Source: CAD feature listing. Evaluate the final solid. Frame: model axes, mm. Face numbers are marked on the shaded views. A direction names the side the tool comes from. Round coordinates to 2 decimals unless told otherwise and drop trailing zeros. Loops run counter-clockwise (first coordinate to the right, second up) from the corner with the lowest first, then second, coordinate; pieces in that order, holes last. Notation, with made-up numbers: (21, 40) - (42, 40) arc R18 cw to (42, 59) - close; hole circle Ø10 at (79.5, 74.25). An arc over 180 degrees is marked (long way). Use CSV: the item, a comma, the result in double quotes. Start each with the question number.
from build123d import *

# Parameters (mm, degrees)
BOSS_EXTRUDE1_DEPTH = 15
SKETCH2_W           = 5.5
SKETCH2_H           = 1.517546376


with BuildPart() as part:
    # Sketch1 → Boss-Extrude1 (new body)
    with BuildSketch(Plane.XY):
        with BuildLine():
            Line((-20, 0), (-20, 23))
            Line((-20, 23), (20, 23))
            Line((20, 23), (20, 0))
            Line((20, 0), (7.5, 0))
            ThreePointArc((7.5, 0), (0, 7.5), (-7.5, 0))
            Line((-7.5, 0), (-20, 0))
        make_face()
    extrude(amount=BOSS_EXTRUDE1_DEPTH)

    # Sketch2 → Cut-Revolve2 (revolve, cut)
    with BuildSketch(Plane(origin=(0, 0, 0), x_dir=(0, 0, -1), z_dir=(1, 0, 0))):
        with Locations((-7.5, 7.241226812)):
            Rectangle(SKETCH2_W, SKETCH2_H)
    revolve(axis=Axis((0, 0, 0), (0, 0, 1)), mode=Mode.SUBTRACT)


solid = part.part
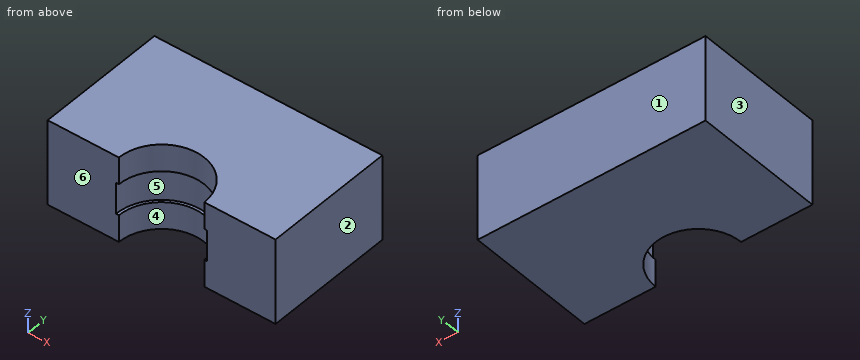
1. Section query D-D on x = 0. Return the cut outline in (y, z).
2. Section query A-A on y = 5.5. Return the cut outline in (x, z).
3. Line query: line 1 along X through (y, z) = (1.5, 12); line 2 along X through (y, z) = (5.5, 6.25); line 3 along Y through (x, z) = (5, 8.75) (3 decimals). Output: solid intervals per line, ascending.
4. Reachability of the marked faces 5 and 6 from +Z, -Z, +X, -X, +Y, -Y: full face, straight path, thin tool, end or side. Return the list, or none.
5. Mould query, pull axis X, two halves, no side actions, for the marked faces 1, 2, 3 and 4. Classes: +X half, -X half, draft (parallel to the pull), parting line (faces both ways), or undercut.
6. Section query C-C on x = 6. Return the cut outline in (y, z).
7. Section query B-B on z = 6. Return the cut outline in (x, y), and give its area (3 significant figures).
Values:
1,outline,"(7.5, 0) - (23, 0) - (23, 15) - (7.5, 15) - (7.5, 10.25) - (8, 10.25) - (8, 4.75) - (7.5, 4.75) - close"
2,outline,"(-20, 0) - (-5.1, 0) - (-5.1, 4.75) - (-5.81, 4.75) - (-5.81, 10.25) - (-5.1, 10.25) - (-5.1, 15) - (-20, 15) - close; (5.1, 0) - (20, 0) - (20, 15) - (5.1, 15) - (5.1, 10.25) - (5.81, 10.25) - (5.81, 4.75) - (5.1, 4.75) - close"
3,line 1,"x = -20 to -7.35, 7.35 to 20"
3,line 2,"x = -20 to -5.81, 5.81 to 20"
3,line 3,"y = 6.245 to 23"
4,face 5,"-Y"
4,face 6,"+Z, -Z, +X, -X, -Y"
5,face 1,"draft"
5,face 2,"+X half"
5,face 3,"-X half"
5,face 4,"undercut"
6,outline,"(4.5, 0) - (23, 0) - (23, 15) - (4.5, 15) - (4.5, 10.25) - (5.29, 10.25) - (5.29, 4.75) - (4.5, 4.75) - close"
7,outline,"(-20, 0) - (-8, 0) arc R8 cw to (8, 0) - (20, 0) - (20, 23) - (-20, 23) - close"
7,area,"819 mm^2"
